The listing builds one solid part. Answer for the finished solid, in the listing's coordinates (mm). A direction names the side the tool comes from. Coordinates: 2 decimals unless noted, no trailing zeros. Order: outer loops, then holes, each group sorted by start corner. A loop starts at its lowest first (then second) coordinate and runs counter-clockwise, first axis right, second up. Notation, with made-up numbers: (37, 25) - (76, 25) arc R30 ccw to (76, 49) - close; hole circle Ø7 at (-39.5, 53.5). An arc over 180 degrees is marked (long way). Use one line per item in the form item = value. Start each with the question number.
Item 1: Section A-A, the plane x = -35.5 is taken. Write down the section's boundary in (y, z), and give its area (3 significant figures).
Item 2: Section C-C, the plane x = 25.4 is taken. Write down the section's boundary in (y, z), and give its area (3 significant figures).
Item 3: Section B-B, the plane y = -13 is taken. Write down the section's boundary in (x, z).
Item 4: Each of these flat-tipped pins is pushed along its axis until it touches: pin 1 Ø8 at (x, y) = (88, -41) entering from +Z; pin 2 Ø5.5 at (x, z) = (54.77, 54.77) entering from -Y; pin 3 Ø21 at (y, z) = (-9, 30) entering from +X. Where does it stop, or does it pass through?
Item 5: The mould has two halves that part along X. Classify faces 1 (the flat face through (50, 1.588, 23)), 2 (the cylindrical face through (21.29, -218.94, 25.04)), 3 (the cylindrical face through (21.339, -217.354, 25.067)): released by +X, released by -X, zero draft, split by the parting line, or undercut.
Item 6: A tool of negligible diameter and unlimited length cuts with its end or side. For faces 4 (the flat face through (49.212, -10, 25)), 5 (the flat face through (0, -9, 25)), 6 (the cylindrical face through (20.44, -79.65, 88.37)), 7 (the flat face through (-18, -85, 1.587)), 8 (the cylindrical face through (18.79, -167.79, 21.91)), from which of +Z, -Z, +X, -X, +Y, -Y can it reach the whole face along a straight path? Write none if from no direction.
Item 7: Consider line 1 along Z through (x, y) = (16, -34); line 2 along Z through (x, y) = (29.5, -113); line 3 along Y through (x, z) = (69, 40). Determine where each line is inside the solid, lowest interval first. Write a range as [from, to].
Item 8: Section D-D, the plane y = -114.5 is taken. Write down the section's boundary in (x, z).
from build123d import *

# Parameters (mm, degrees)
F1_DEPTH = 50.8
F2_R     = 38.1
F3_DEPTH = 76.2
F4_R     = 50.8
F5_DEPTH = 44.45
F6_T     = -1.5875
F7_W     = 66.675
F7_H     = 66.675
F7_R     = 2.15265
F7_W_2   = 47.625
F7_H_2   = 47.625
F8_DEPTH = 1.5875


with BuildPart() as f1:
    # F0 (on Top) → F1 (new body)
    with BuildSketch(Plane.XY):
        with BuildLine():
            Line((50.8, 0), (0, 0))
            Line((0, 0), (0, -19.05))
            ThreePointArc((0, -19.05), (25.4, -219.0237769937), (50.8, -19.05))
            Line((50.8, -19.05), (50.8, 0))
        make_face()
    extrude(amount=F1_DEPTH)

    # F2 (on face) → F3 (join)
    with BuildSketch(Plane.XY.offset(50.8)):
        with Locations((25.4, -117.4237769937)):
            Circle(F2_R)
    extrude(amount=F3_DEPTH)

    # F4 (on face) → F5 (cut)
    with BuildSketch(Plane(origin=(0, 0, 0), x_dir=(1, 0, 0), z_dir=(0, 0, -1))):
        with Locations((25.4, 117.4237769937)):
            Circle(F4_R)
    extrude(amount=-F5_DEPTH, mode=Mode.SUBTRACT)

    # F6
    f6_openings = [f1.faces().sort_by_distance(p)[0] for p in [
        (25.4, 0, 25.4),
    ]]
    offset(amount=F6_T, openings=f6_openings, kind=Kind.INTERSECTION)

    # F7 (on face) → F8 (join)
    with BuildSketch(Plane(origin=(0, 0, 0), x_dir=(-1, 0, 0), z_dir=(0, 1, 0))):
        with Locations((-25.4, 25.4)):
            Rectangle(F7_W, F7_H)
        with Locations((-54.76875, -3.96875)):
            Circle(F7_R, mode=Mode.SUBTRACT)
        with Locations((3.96875, -3.96875)):
            Circle(F7_R, mode=Mode.SUBTRACT)
        with Locations((-54.76875, 54.76875)):
            Circle(F7_R, mode=Mode.SUBTRACT)
        with Locations((-25.4, 25.4)):
            Rectangle(F7_W_2, F7_H_2, mode=Mode.SUBTRACT)
        with Locations((3.96875, 54.76875)):
            Circle(F7_R, mode=Mode.SUBTRACT)
    extrude(amount=F8_DEPTH)


solid = f1.part
Response:
q1.outline = (-198.75, 0) - (-36.1, 0) - (-36.1, 50.8) - (-198.75, 50.8) - close; hole (-196.76, 1.59) - (-38.09, 1.59) - (-38.09, 49.21) - (-196.76, 49.21) - close
q1.area = 706 mm2
q2.outline = (-219.02, 0) - (-168.22, 0) - (-168.22, 44.45) - (-66.62, 44.45) - (-66.62, 0) - (0, 0) - (0, -7.94) - (1.59, -7.94) - (1.59, 1.59) - (-65.04, 1.59) - (-65.04, 46.04) - (-169.81, 46.04) - (-169.81, 1.59) - (-217.44, 1.59) - (-217.44, 49.21) - (-153.94, 49.21) - (-153.94, 125.41) - (-80.91, 125.41) - (-80.91, 49.21) - (1.59, 49.21) - (1.59, 58.74) - (0, 58.74) - (0, 50.8) - (-79.32, 50.8) - (-79.32, 127) - (-155.52, 127) - (-155.52, 50.8) - (-219.02, 50.8) - close
q2.area = 1,180 mm2
q3.outline = (0, 0) - (50.8, 0) - (50.8, 50.8) - (0, 50.8) - close; hole (1.59, 1.59) - (49.21, 1.59) - (49.21, 49.21) - (1.59, 49.21) - close
q4.pin_1 = 50.8
q4.pin_2 = -144.68
q4.pin_3 = 58.74
q5.face_1 = zero draft
q5.face_2 = split by the parting line
q5.face_3 = undercut
q6.face_4 = +Y
q6.face_5 = +Z, -Z, -X
q6.face_6 = +Z
q6.face_7 = none
q6.face_8 = -Z
q7.line_1 = [0, 1.59], [49.21, 50.8]
q7.line_2 = [44.45, 46.04], [125.41, 127]
q7.line_3 = [-209.19, -207.43], [-146.47, -143.49], [-91.35, -88.38], [-27.42, -25.65]
q8.outline = (-76.16, 0) - (-25.32, 0) - (-25.32, 44.45) - (76.12, 44.45) - (76.12, 0) - (126.96, 0) - (126.96, 50.8) - (63.39, 50.8) - (63.39, 127) - (-12.59, 127) - (-12.59, 50.8) - (-76.16, 50.8) - close; hole (-74.57, 1.59) - (-26.91, 1.59) - (-26.91, 46.04) - (77.71, 46.04) - (77.71, 1.59) - (125.37, 1.59) - (125.37, 49.21) - (61.8, 49.21) - (61.8, 125.41) - (-11, 125.41) - (-11, 49.21) - (-74.57, 49.21) - close
